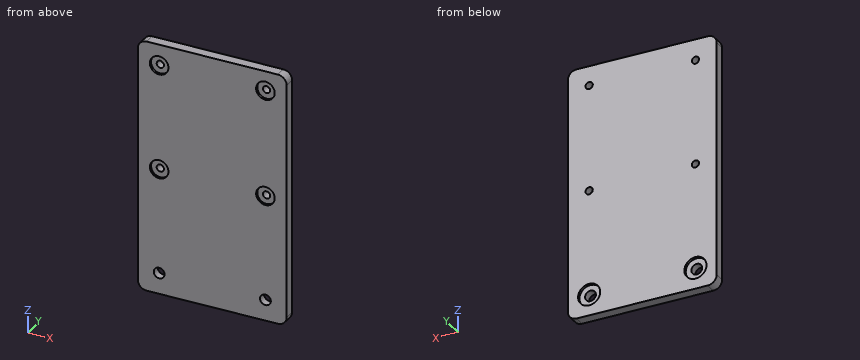
from build123d import *

# Parameters (mm, degrees)
EXTRUDE_1_DEPTH     = 6
SKETCH_2_R          = 2.05
SKETCH_2_R_2        = 3.05
CUT_EXTRUDE_1_DEPTH = 6
SKETCH_3_R          = 5.25
CUT_EXTRUDE_2_DEPTH = 1.3
SKETCH_5_R          = 6.25
CUT_EXTRUDE_3_DEPTH = 1.5


with BuildPart() as part:
    # 草图1 → 凸台-拉伸1 (new body)
    with BuildSketch(Plane(origin=(0, 0, 0), x_dir=(1, 0, 0), z_dir=(0, 1, 0))):
        with BuildLine():
            Line((37, -72), (-37, -72))
            ThreePointArc((-37, -72), (-40.535533906, -70.535533906), (-42, -67))
            Line((-42, -67), (-42, 67))
            ThreePointArc((-42, 67), (-40.535533906, 70.535533906), (-37, 72))
            Line((-37, 72), (37, 72))
            ThreePointArc((37, 72), (40.535533906, 70.535533906), (42, 67))
            Line((42, 67), (42, -67))
            ThreePointArc((42, -67), (40.535533906, -70.535533906), (37, -72))
        make_face()
    extrude(amount=EXTRUDE_1_DEPTH)

    # 草图2 → 切除-拉伸1 (cut)
    with BuildSketch(Plane.XZ):
        with Locations(Location((-30, 60, 0), (0, 0, 270))):
            Circle(SKETCH_2_R)
        with Locations(Location((30, 60.83466259, 0), (0, 0, 270))):
            Circle(SKETCH_2_R)
        with Locations(Location((-30, 0, 0), (0, 0, 270))):
            Circle(SKETCH_2_R)
        with Locations(Location((30, 0, 0), (0, 0, 270))):
            Circle(SKETCH_2_R)
        with Locations(Location((-30, -60, 0), (0, 0, 270))):
            Circle(SKETCH_2_R_2)
        with Locations(Location((30, -60, 0), (0, 0, 270))):
            Circle(SKETCH_2_R_2)
    extrude(amount=-CUT_EXTRUDE_1_DEPTH, mode=Mode.SUBTRACT)

    # 草图3 → 切除-拉伸2 (cut)
    with BuildSketch(Plane.XZ):
        with Locations(Location((-30, 60, 0), (0, 0, 270))):
            Circle(SKETCH_3_R)
        with Locations(Location((30, 60.83466259, 0), (0, 0, 270))):
            Circle(SKETCH_3_R)
        with Locations(Location((-30, 0, 0), (0, 0, 270))):
            Circle(SKETCH_3_R)
        with Locations(Location((30, 0, 0), (0, 0, 270))):
            Circle(SKETCH_3_R)
    extrude(amount=-CUT_EXTRUDE_2_DEPTH, mode=Mode.SUBTRACT)

    # 草图5 → 切除-拉伸3 (cut)
    with BuildSketch(Plane(origin=(0, 6, 0), x_dir=(1, 0, 0), z_dir=(0, 1, 0))):
        with Locations(Location((-30, 60, 0), (0, 0, 270))):
            Circle(SKETCH_5_R)
        with Locations(Location((30, 60, 0), (0, 0, 270))):
            Circle(SKETCH_5_R)
    extrude(amount=-CUT_EXTRUDE_3_DEPTH, mode=Mode.SUBTRACT)


solid = part.part
Verification items for the finished model (mm, model axes). Give positions to 0.01 mm unless a question says otherwise; leave off trailing zeros. Write each loop counter-clockwise with the first axis right and the second up, starting at its lowest first coordinate (ties: lowest second). Pieces come first, ordered by that corner, then holes.
(1) Material ranges on line 1 (X direction, y = 5.45, z = -60); line 2 (X direction, y = 3.75, z = 0); line 3 (Z direction, x = 31.5, y = 4.3), recorded low to high.
(2) Gauge pin test, flat ends, axial feed: pin 1 (5 mm diameter, centred on x = -30, z = 0, fed in from -Y); pin 2 (10 mm diameter, centred on x = 30, z = -60, fed in from +Y). Record the tip position at first contact, or that the pin passes through.
(3) Cross-section at A-A (x = -30). Enter the section's corners in (y, z), plus the area to 3 significant figures.
(4) Cross-section at B-B (z = 0). Enter the section's corners in (x, y).
Worked out:
1. line 1: x = -42 to -36.25, -23.75 to 23.75, 36.25 to 42
1. line 2: x = -42 to -32.05, -27.95 to 27.95, 32.05 to 42
1. line 3: z = -72 to -62.66, -57.34 to -1.4, 1.4 to 59.44, 62.23 to 72
2. pin 1: stops at y = 1.3
2. pin 2: stops at y = 4.5
3. outline: (0, -72) - (6, -72) - (6, -66.25) - (4.5, -66.25) - (4.5, -63.05) - (0, -63.05) - close; (0, -56.95) - (4.5, -56.95) - (4.5, -53.75) - (6, -53.75) - (6, -2.05) - (1.3, -2.05) - (1.3, -5.25) - (0, -5.25) - close; (0, 5.25) - (1.3, 5.25) - (1.3, 2.05) - (6, 2.05) - (6, 57.95) - (1.3, 57.95) - (1.3, 54.75) - (0, 54.75) - close; (0, 65.25) - (1.3, 65.25) - (1.3, 62.05) - (6, 62.05) - (6, 72) - (0, 72) - close
3. area: 752 mm2
4. outline: (-42, 0) - (-35.25, 0) - (-35.25, 1.3) - (-32.05, 1.3) - (-32.05, 6) - (-42, 6) - close; (-27.95, 1.3) - (-24.75, 1.3) - (-24.75, 0) - (24.75, 0) - (24.75, 1.3) - (27.95, 1.3) - (27.95, 6) - (-27.95, 6) - close; (32.05, 1.3) - (35.25, 1.3) - (35.25, 0) - (42, 0) - (42, 6) - (32.05, 6) - close
